Here's the drawing with two shaded views (mm, measured from the low corner). I have some questions. A direction names the side the tool comes from. Coordinates: 2 decimals unless noted, no trailing zeros. Loops run counter-clockwise (first coordinate to the right, second up) from the corner with the lowest first, then second, coordinate; pieces in that order, holes last.
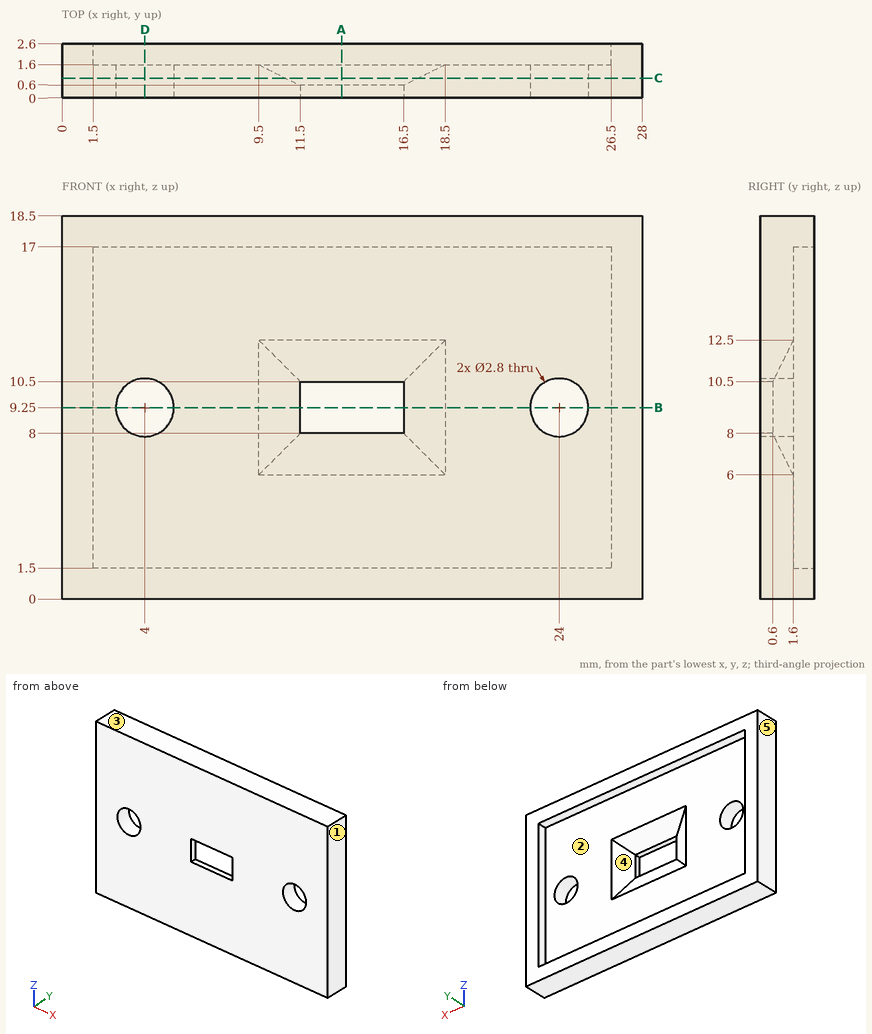
Q1. Suppose I cut it at C-C on y = 0.95. Write out the boundary of the cut face in (x, z).
Q2. We'd pull the mould along Z, two halves only. Please class the marked faces 3, 4 and 5: pulls with the +Z half, pulls with the -Z half, needs draft (parallel to the pull), parting line crosses it, or undercut.
Q3. Suppose I cut it at B-B on z = 9.25. Write out the boundary of the cut face in (x, y), and give its area (3 significant figures).
Q4. For the marked faces 1 and 2, which set-ups out of +Z, -Z, +X, -X, +Y, -Y let a thin tool reach every point of the face, with its end or its side?
Q5. Suppose I cut it at A-A on x = 13.5. Write out the boundary of the cut face in (y, z), and give its area (3 significant figures).
Q6. Suppose I cut it at D-D on x = 4. Write out the boundary of the cut face in (y, z), and give its area (3 significant figures).
Q7. Please list where these lines run through material, in increasing order: probe 1 along X at (y, z) = (0.55, 9.25); probe 2 along X at (y, z) = (1.3, 9.25); probe 3 along X at (y, z) = (1.9, 15).
Q8. Will this pin go through, and if not, where does the flat tip stop? P1, Ø4.5, axis at x = 4, z = 9.25, coming from the +Y side.
Check values:
1. outline: (0, 0) - (28, 0) - (28, 18.5) - (0, 18.5) - close; hole circle Ø2.8 at (4, 9.25); hole (10.8, 7.3) - (17.2, 7.3) - (17.2, 11.2) - (10.8, 11.2) - close; hole circle Ø2.8 at (24, 9.25)
2. face 3: pulls with the +Z half
2. face 4: undercut
2. face 5: needs draft
3. outline: (0, 0) - (2.6, 0) - (2.6, 1.6) - (1.5, 1.6) - (1.5, 2.6) - (0, 2.6) - close; (5.4, 0) - (11.5, 0) - (11.5, 0.6) - (9.5, 1.6) - (5.4, 1.6) - close; (16.5, 0) - (22.6, 0) - (22.6, 1.6) - (18.5, 1.6) - (16.5, 0.6) - close; (25.4, 0) - (28, 0) - (28, 2.6) - (26.5, 2.6) - (26.5, 1.6) - (25.4, 1.6) - close
3. area: 28.8 mm2
4. face 1: +Z, -Z, +X, +Y, -Y
4. face 2: +Y
5. outline: (0, 0) - (2.6, 0) - (2.6, 1.5) - (1.6, 1.5) - (1.6, 6) - (0.6, 8) - (0, 8) - close; (0, 10.5) - (0.6, 10.5) - (1.6, 12.5) - (1.6, 17) - (2.6, 17) - (2.6, 18.5) - (0, 18.5) - close
5. area: 26.6 mm2
6. outline: (0, 0) - (2.6, 0) - (2.6, 1.5) - (1.6, 1.5) - (1.6, 7.85) - (0, 7.85) - close; (0, 10.65) - (1.6, 10.65) - (1.6, 17) - (2.6, 17) - (2.6, 18.5) - (0, 18.5) - close
6. area: 28.1 mm2
7. probe 1: x = 0 to 2.6, 5.4 to 11.5, 16.5 to 22.6, 25.4 to 28
7. probe 2: x = 0 to 2.6, 5.4 to 10.1, 17.9 to 22.6, 25.4 to 28
7. probe 3: x = 0 to 1.5, 26.5 to 28
8. P1: stops at y = 1.6
